```python
from build123d import *

# Parameters (mm, degrees)
SKETCH1_W                 = 85.5
SKETCH1_H                 = 127.8
BOSS_EXTRUDE1_DEPTH       = 9
TAP_DRILL_FOR_6_32_TAP1_D = 2.7051
LPATTERN1_COUNT           = 3
LPATTERN1_PITCH           = 59.9
MIRROR1_COPY_1_D          = 2.7051
MIRROR1_COPY_2_D          = 2.7051


with BuildPart() as part:
    # Sketch1 → Boss-Extrude1 (new body)
    with BuildSketch(Plane(origin=(0, 0, 0), x_dir=(1, 0, 0), z_dir=(0, 1, 0))):
        with Locations((42.75, 63.9)):
            Rectangle(SKETCH1_W, SKETCH1_H)
    extrude(amount=BOSS_EXTRUDE1_DEPTH)

    # Tap Drill for #6-32 Tap1 (through all)
    with Locations(Plane(origin=(0, 9, 0), x_dir=(1, 0, 0), z_dir=(0, 1, 0))):
        with Locations((82.5, 4)):
            tap_drill_for_6_32_tap1 = Hole(TAP_DRILL_FOR_6_32_TAP1_D / 2)

    # LPattern1: Tap Drill for #6-32 Tap1 ×3
    with Locations(*[(0, 0, -i * LPATTERN1_PITCH) for i in range(1, LPATTERN1_COUNT)]):
        add(tap_drill_for_6_32_tap1, mode=Mode.SUBTRACT)

    # Mirror1: Tap Drill for #6-32 Tap1 across plane
    add(tap_drill_for_6_32_tap1.mirror(Plane(origin=(42.75, 0, 0), x_dir=(0, 0, 1), z_dir=(1, 0, 0))), mode=Mode.SUBTRACT)

    # Mirror1 copy 1 (through all)
    with Locations(Plane(origin=(85.5, 9, -59.9), x_dir=(-1, 0, 0), z_dir=(0, 1, 0))):
        with Locations((82.5, -4)):
            Hole(MIRROR1_COPY_1_D / 2)

    # Mirror1 copy 2 (through all)
    with Locations(Plane(origin=(85.5, 9, -119.8), x_dir=(-1, 0, 0), z_dir=(0, 1, 0))):
        with Locations((82.5, -4)):
            Hole(MIRROR1_COPY_2_D / 2)


solid = part.part
```
Part model, mm, in its own coordinate system. Round coordinates to 2 decimals unless told otherwise and drop trailing zeros. Loops run counter-clockwise (first coordinate to the right, second up) from the corner with the lowest first, then second, coordinate; pieces in that order, holes last.
1. Drill centre lines: line 1 along Z through (x, y) = (82.5, 3); line 2 along X through (y, z) = (6, -123.8). Where is each one in solid material? Low to high.
Solutions:
line 1: z = -127.8 to -125.15, -122.45 to -65.25, -62.55 to -5.35, -2.65 to 0
line 2: x = 0 to 1.65, 4.35 to 81.15, 83.85 to 85.5
2. Slice it at A-A (x = 3). Give the cut face in (y, z).
Solutions:
outline: (0, -127.8) - (9, -127.8) - (9, -125.15) - (0, -125.15) - close; (0, -122.45) - (9, -122.45) - (9, -65.25) - (0, -65.25) - close; (0, -62.55) - (9, -62.55) - (9, -5.35) - (0, -5.35) - close; (0, -2.65) - (9, -2.65) - (9, 0) - (0, 0) - close
3. Flat gauge pin, fed straight in: pin 1 (2 mm diameter, centred on x = 82.5, z = -123.8, fed in from -Y). Where does the tip first touch, or does it go through?
Solutions:
pin 1: passes through
4. Slice it at B-B (z = -123.8). Give the cut face in (x, y), and give its area (3 significant figures).
Solutions:
outline: (0, 0) - (1.65, 0) - (1.65, 9) - (0, 9) - close; (4.35, 0) - (81.15, 0) - (81.15, 9) - (4.35, 9) - close; (83.85, 0) - (85.5, 0) - (85.5, 9) - (83.85, 9) - close
area: 721 mm2
5. Two-plate mould, pull along X, no slides. Class faces 1 (the face through (42, 9, -65)), 2 (the face through (2.82, 4.44, -122.46)), 3 (the face through (4.25, 4.44, -3.48)), 4 (the face through (85.5, 4, -63)): pulls with the +X half, pulls with the -X half, needs draft (parallel to the pull), parting line crosses it, or undercut.
Solutions:
face 1: needs draft
face 2: undercut
face 3: undercut
face 4: pulls with the +X half
